The model under review builds one solid part; all positions refer to its coordinate system, in mm. Face numbers are marked on the shaded views. A direction names the side the tool comes from. Coordinates: 2 decimals unless noted, no trailing zeros. Write each loop counter-clockwise with the first axis right and the second up, starting at its lowest first coordinate (ties: lowest second). Pieces come first, ordered by that corner, then holes. Notation, with made-up numbers: (76, 37) - (133, 37) arc R36 cw to (133, 75) - close; hole circle Ø6 at (-10, -11.75). An arc over 180 degrees is marked (long way). Answer as CSV lines item,"result". Start each with the question number.
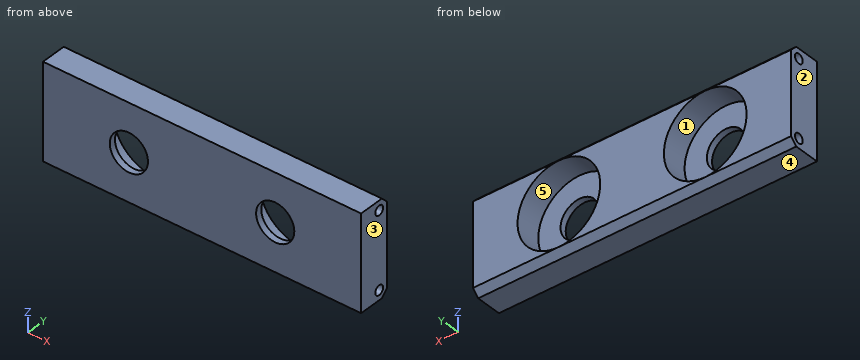
```python
from build123d import *

# Parameters (mm, degrees)
SKETCH1_W           = 100
SKETCH1_H           = 30
BOSS_EXTRUDE1_DEPTH = 6
SKETCH2_R           = 6
CUT_EXTRUDE1_DEPTH  = 105.575331699
CHAMFER1_SIZE       = 2
SKETCH3_R           = 1.5
CUT_EXTRUDE2_DEPTH  = 7
CUT_EXTRUDE3_START  = -7
SKETCH4_R           = 1.5
CUT_EXTRUDE3_DEPTH  = 7
SKETCH5_W           = 100
SKETCH5_H           = 30
SKETCH5_R           = 6
BOSS_EXTRUDE2_DEPTH = 4
SKETCH6_R           = 13
CUT_EXTRUDE4_DEPTH  = 8


with BuildPart() as part:
    # Sketch1 → Boss-Extrude1 (new body)
    with BuildSketch(Plane(origin=(0, 0, 0), x_dir=(1, 0, 0), z_dir=(0, 1, 0))):
        with Locations((50, 15)):
            Rectangle(SKETCH1_W, SKETCH1_H)
    extrude(amount=BOSS_EXTRUDE1_DEPTH)

    # Sketch2 → Cut-Extrude1 (cut, through all)
    with BuildSketch(Plane(origin=(0, 6, 0), x_dir=(1, 0, 0), z_dir=(0, 1, 0))):
        with Locations(Location((27, 15, 0), (0, 0, 270))):
            Circle(SKETCH2_R)
        with Locations(Location((73, 15, 0), (0, 0, 270))):
            Circle(SKETCH2_R)
    extrude(amount=-CUT_EXTRUDE1_DEPTH, mode=Mode.SUBTRACT)

    # Chamfer1
    chamfer1_edges = [part.edges().sort_by_distance(p)[0] for p in [
        (50, 6, -30),
        (50, 6, 0),
    ]]
    chamfer(chamfer1_edges, length=CHAMFER1_SIZE)

    # Sketch3 → Cut-Extrude2 (cut)
    with BuildSketch(Plane(origin=(100, 0, 0), x_dir=(0, 0, -1), z_dir=(1, 0, 0))):
        with Locations((3, 3)):
            Circle(SKETCH3_R)
        with Locations((27, 3)):
            Circle(SKETCH3_R)
    extrude(amount=-CUT_EXTRUDE2_DEPTH, mode=Mode.SUBTRACT)

    # Sketch4 → Cut-Extrude3 (cut)
    with BuildSketch(Plane.ZY.offset(CUT_EXTRUDE3_START)):
        with Locations(Location((-27, 3, 0), (0, 0, 180))):
            Circle(SKETCH4_R)
        with Locations(Location((-3, 3, 0), (0, 0, 180))):
            Circle(SKETCH4_R)
    extrude(amount=CUT_EXTRUDE3_DEPTH, mode=Mode.SUBTRACT)

    # Sketch5 → Boss-Extrude2 (add)
    with BuildSketch(Plane.XZ):
        with Locations((50, -15)):
            Rectangle(SKETCH5_W, SKETCH5_H)
        with Locations(Location((27, -15, 0), (0, 0, 90))):
            Circle(SKETCH5_R, mode=Mode.SUBTRACT)
        with Locations(Location((73, -15, 0), (0, 0, 90))):
            Circle(SKETCH5_R, mode=Mode.SUBTRACT)
    extrude(amount=BOSS_EXTRUDE2_DEPTH)

    # Sketch6 → Cut-Extrude4 (cut)
    with BuildSketch(Plane(origin=(0, 6, 0), x_dir=(1, 0, 0), z_dir=(0, 1, 0))):
        with Locations(Location((27, 15, 0), (0, 0, 270))):
            Circle(SKETCH6_R)
        with Locations(Location((73, 15, 0), (0, 0, 270))):
            Circle(SKETCH6_R)
    extrude(amount=-CUT_EXTRUDE4_DEPTH, mode=Mode.SUBTRACT)


solid = part.part
```
(1) The part is to be moulded in two halves that separate along X. For the marked faces 3, 4 and 5, say which applies: released by +X, released by -X, zero draft, split by the parting line, or undercut.
(2) Add section D-D on z = -13. Give the boundary of the cut face in (x, y).
(3) Wall thickness on line 1 (X direction, y = 3.75, z = -15); line 2 (Z direction, x = 3, y = 3); line 3 (Y direction, x = 2, z = -3): over which ranges is each line inside the solid? List them lowest first.
(4) For the marked faces 1 and 2, list the 3-axis set-ups (+Z, -Z, +X, -X, +Y, -Y) from which the entire face can be reached by the end or side of a thin tool; tool diameter is ignored.
(5) For pin 1 (8 mm diameter, centred on x = 72.5, z = -18.5, fed in from +Y); pin 2 (1.5 mm diameter, centred on y = 2.5, z = -27, fed in from +X); pin 3 (1.8 mm diameter, centred on y = 3, z = -27, fed in from -X), all flat-tipped, find the tip position at first contact; note any pin that passes through.
(6) Add section C-C on x = 75. Give the boundary of the cut face in (y, z).
(7) Add section A-A on y = 3. Give the boundary of the cut face in (x, z), then the cut area to 3 significant figures.
(8) Add section B-B on z = -3. Give the boundary of the cut face in (x, y).
Reported:
1,face 3,"released by +X"
1,face 4,"zero draft"
1,face 5,"undercut"
2,outline,"(0, -4) - (21.34, -4) - (21.34, -2) - (14.15, -2) - (14.15, 6) - (0, 6) - close; (32.66, -4) - (67.34, -4) - (67.34, -2) - (60.15, -2) - (60.15, 6) - (39.85, 6) - (39.85, -2) - (32.66, -2) - close; (78.66, -4) - (100, -4) - (100, 6) - (85.85, 6) - (85.85, -2) - (78.66, -2) - close"
3,line 1,"0 to 14, 40 to 60, 86 to 100"
3,line 2,"-30 to -28.5, -25.5 to -4.5, -1.5 to 0"
3,line 3,"-4 to 1.5, 4.5 to 6"
4,face 1,"+Y"
4,face 2,"+Z, -Z, -X, +Y, -Y"
5,pin 1,"y = -2"
5,pin 2,"x = 93"
5,pin 3,"x = 7"
6,outline,"(-4, -30) - (4, -30) - (6, -28) - (6, -27.85) - (-2, -27.85) - (-2, -20.66) - (-4, -20.66) - close; (-4, -9.34) - (-2, -9.34) - (-2, -2.15) - (6, -2.15) - (6, -2) - (4, 0) - (-4, 0) - close"
7,outline,"(0, -30) - (100, -30) - (100, -28.5) - (93, -28.5) - (93, -25.5) - (100, -25.5) - (100, -4.5) - (93, -4.5) - (93, -1.5) - (100, -1.5) - (100, 0) - (0, 0) - (0, -1.5) - (7, -1.5) - (7, -4.5) - (0, -4.5) - (0, -25.5) - (7, -25.5) - (7, -28.5) - (0, -28.5) - close; hole circle Ø26 at (27, -15); hole circle Ø26 at (73, -15)"
7,area,"1,850 mm²"
8,outline,"(0, -4) - (100, -4) - (100, 1.5) - (93, 1.5) - (93, 4.5) - (100, 4.5) - (100, 6) - (78, 6) - (78, -2) - (68, -2) - (68, 6) - (32, 6) - (32, -2) - (22, -2) - (22, 6) - (0, 6) - (0, 4.5) - (7, 4.5) - (7, 1.5) - (0, 1.5) - close"
